Geometry check sheet. Reference: the model listing, model coordinates, mm. Face numbers are marked on the shaded views. A direction names the side the tool comes from. Round coordinates to 2 decimals unless told otherwise and drop trailing zeros. Write each loop counter-clockwise with the first axis right and the second up, starting at its lowest first coordinate (ties: lowest second). Pieces come first, ordered by that corner, then holes. Notation, with made-up numbers: M -14.75,5 L 23.25,5 A19 cw 23.25,25 Z; hole C 31,19.5 d9. An arc over 180 degrees is marked long. Use a Markdown table: item, result.
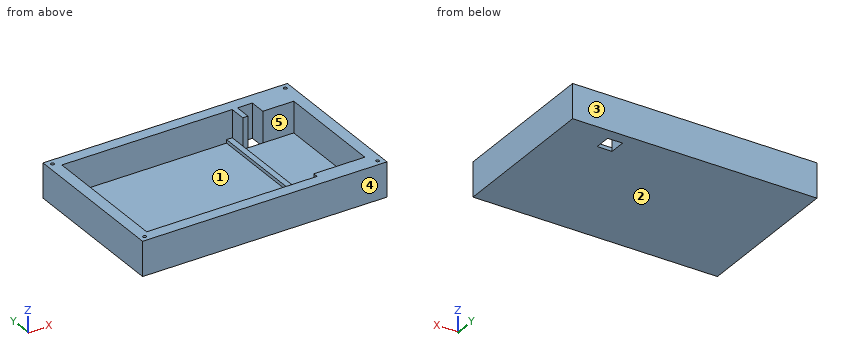
Autodesk Fusion 360 part; units mm, degrees
sketch "Sketch1" plane through (0, 0, 0) normal (0, 0, 1) x (1, 0, 0)
  line L0 (-50, 40) -> (143.2, 40)
  line L1 (143.2, 40) -> (143.2, -75.2)
  line L2 (143.2, -75.2) -> (-50, -75.2)
  line L3 (-50, -75.2) -> (-50, 40)
  line L4 (-60, 50) -> (153.2, 50)
  line L5 (153.2, 50) -> (153.2, -85.2)
  line L6 (153.2, -85.2) -> (-60, -85.2)
  line L7 (-60, -85.2) -> (-60, 50)
  circle A0 centre (-55, 45) radius 1.45
  circle A1 centre (148.2, 45) radius 1.45
  circle A2 centre (148.2, -80.2) radius 1.45
  circle A3 centre (-55, -80.2) radius 1.45
  line L8 (143.2, -75.2) -> (98.7, -75.2)
  line L9 (98.7, -75.2) -> (98.7, 21.3)
  line L10 (98.7, 21.3) -> (143.2, 21.3)
  line L11 (143.2, 21.3) -> (143.2, -75.2)
  line L12 (98.7, 21.3) -> (143.2, 21.3)
  line L13 (143.2, 21.3) -> (143.2, 40)
  line L14 (143.2, 40) -> (98.7, 40)
  line L15 (98.7, 40) -> (98.7, 21.3)
  line L16 (98.7, 40) -> (93.7, 40)
  line L17 (93.7, 40) -> (93.7, -75.2)
  line L18 (93.7, -75.2) -> (98.7, -75.2)
  line L19 (98.7, -75.2) -> (98.7, 40)
  dimension "d1" = 193.2
  dimension "d2" = 115.2
  dimension "d3" = 213.2
  dimension "d4" = 135.2
  dimension "d5" = 10
  dimension "d6" = 10
  dimension "d7" = 2.9
  dimension "d8" = 5
  dimension "d9" = 5
  dimension "d10" = 2.9
  dimension "d11" = 5
  dimension "d12" = 5
  dimension "d13" = 2.9
  dimension "d14" = 5
  dimension "d15" = 5
  dimension "d16" = 2.9
  dimension "d17" = 5
  dimension "d18" = 5
  dimension "d19" = 44.5
  dimension "d20" = 96.5
  dimension "d21" = 5
extrude "Extrude1" add sketch "Sketch1" along normal blind 3 contours L0 L2 L3 L17 | L1 L2 L8 L9 L10 L11 L12 L19 makes body 1 at (113.5333, -43.0333, 0) makes body 2 at (-2.1, 1.6, 0)
extrude "Extrude2" add sketch "Sketch1" along normal blind 6 contours L0 L2 L9 L15 L16 L17 L18 L19 bodies 1 2
extrude "Extrude3" add sketch "Sketch1" along normal blind 3 separate body contours A0 | A1 | A2 | A3 makes body 3 at (149.5361, -79.6368, 2) makes body 4 at (-54.0406, -79.1128, 2) makes body 5 at (149.3558, 45.8755, 2) makes body 6 at (-56.4213, 45.2873, 2)
extrude "Extrude4" add sketch "Sketch1" along normal blind 30 contours L0 L1 L10 L12 L13 L14 L15 L19 | L4 L5 L6 L7 bodies 1 3 4 5 6
sketch "Sketch2" plane through (0, 21.3, 0) normal (0, -1, 0) x (1, 0, 0)
  line L0 (98.7, 3) -> (143.2, 3)
  line L1 (143.2, 3) -> (143.2, 30)
  line L2 (143.2, 30) -> (98.7, 30)
  line L3 (98.7, 30) -> (98.7, 6)
  line L4 (98.7, 6) -> (98.7, 3)
  line L5 (103.2, 30) -> (116.2, 30)
  line L6 (116.2, 30) -> (116.2, 3)
  line L7 (116.2, 3) -> (103.2, 3)
  line L8 (103.2, 3) -> (103.2, 30)
  dimension "d30" = 13
  dimension "d32" = 4.5
extrude "Extrude5" cut sketch "Sketch2" against normal blind 18.7 contours L0 L2 L5 L6 L7 L8 bodies 1
sketch "Sketch3" plane through (0, 0, 3) normal (0, 0, 1) x (-1, 0, 0)
  line L0 (-98.7, 75.2) -> (-143.2, 75.2)
  line L1 (-143.2, 75.2) -> (-143.2, -21.3)
  line L2 (-143.2, -21.3) -> (-116.2, -21.3)
  line L3 (-116.2, -21.3) -> (-116.2, -40)
  line L4 (-116.2, -40) -> (-103.2, -40)
  line L5 (-103.2, -40) -> (-103.2, -21.3)
  line L6 (-103.2, -21.3) -> (-98.7, -21.3)
  line L7 (-98.7, -21.3) -> (-98.7, 75.2)
  line L8 (-103.2, -40) -> (-116.2, -40)
  line L9 (-116.2, -40) -> (-116.2, -21.3)
  line L10 (-116.2, -21.3) -> (-103.2, -21.3)
  line L11 (-103.2, -21.3) -> (-103.2, -40)
extrude "Extrude6" cut sketch "Sketch3" against normal blind 6 contours L3 L4 L5 L8 L9 L10 L11 bodies 1
sketch "Sketch4" plane through (0, -75.2, 0) normal (0, 1, 0) x (-1, 0, 0)
  line L0 (-143.2, 3) -> (-98.7, 3)
  line L1 (-98.7, 3) -> (-98.7, 6)
  line L2 (-98.7, 6) -> (-93.7, 6)
  line L3 (-93.7, 6) -> (-93.7, 3)
  line L4 (-93.7, 3) -> (50, 3)
  line L5 (50, 3) -> (50, 30)
  line L6 (50, 30) -> (-143.2, 30)
  line L7 (-143.2, 30) -> (-143.2, 3)
  line L8 (-98.7, 3) -> (-143.2, 3)
  line L9 (-143.2, 3) -> (-143.2, 30)
  line L10 (-143.2, 30) -> (-98.7, 30)
  line L11 (-98.7, 30) -> (-98.7, 3)
extrude "Extrude7" add sketch "Sketch4" along normal blind 4.5 contours L0 L1 L6 L7 L8 L9 L10 L11 bodies 1
extrude "Extrude8" cut 2 faces at (101.7, 21.3, 13) (125.2, 21.3, 12) along direction (0, 1, 0) blind 4.5 on bodies 1 bodies 1
extrude "Extrude9" add 1 faces at (111.8667, 21.3, 2) along direction (0, 1, 0) blind 4.5 on bodies 1 bodies 1
equation "d3 = 193.2 mm + 20 mm"
equation "d4 = 115.2 mm + 20 mm"
Item 1: Cross-section at A-A, the plane y = 37. Record the cut outline in (x, z).
Outcome:
| item | result |
|---|---|
| outline | M -60,0 L 103.2,0 L 103.2,30 L 98.7,30 L 98.7,6 L 93.7,6 L 93.7,3 L -50,3 L -50,30 L -60,30 Z; M 116.2,0 L 153.2,0 L 153.2,30 L 116.2,30 Z |
Item 2: Cross-section at C-C, the plane z = 13. Record the cut outline in (x, y), and give its area (3 significant figures).
Outcome:
| item | result |
|---|---|
| outline | M -60,-85.2 L 153.2,-85.2 L 153.2,50 L -60,50 Z; hole C -55,-80.2 d2.9; hole C -55,45 d2.9; hole M -50,-75.2 L 98.7,-75.2 L 98.7,-70.7 L 143.2,-70.7 L 143.2,25.8 L 116.2,25.8 L 116.2,40 L 103.2,40 L 103.2,25.8 L 98.7,25.8 L 98.7,40 L -50,40 Z; hole C 148.2,-80.2 d2.9; hole C 148.2,45 d2.9 |
| area | 7,190 mm2 |
Item 3: Cross-section at B-B, the plane x = 96. Record the cut outline in (y, z).
Outcome:
| item | result |
|---|---|
| outline | M -85.2,0 L 50,0 L 50,30 L 40,30 L 40,6 L -75.2,6 L -75.2,30 L -85.2,30 Z |
Item 4: Access from +Z, -Z, +X, -X, +Y, -Y to the whole of each face (thin tool, end or side, straight path). Record for the marked faces 1 and 2.
Outcome:
| item | result |
|---|---|
| face 1 | +Z |
| face 2 | -Z, +X, -X, +Y, -Y |
Item 5: Mould release check, pull along Y, two halves, no side actions. Record for the marked faces 3, 4 and 5: +Y half, -Y half, draft (parallel to the pull), parting line (faces both ways), or undercut.
Outcome:
| item | result |
|---|---|
| face 3 | +Y half |
| face 4 | -Y half |
| face 5 | undercut |
Item 6: Go/stop test with flat-tipped pins: pin 1 (4 mm diameter, centred on x = 44, y = -41, fed in from +Z); pin 2 (4 mm diameter, centred on x = 96.5, y = 3.5, fed in from +Z). Record where each tip stops, or that it passes through.
Outcome:
| item | result |
|---|---|
| pin 1 | stops at z = 3 |
| pin 2 | stops at z = 6 |
Item 7: Cross-section at D-D, the plane y = -66. Record the cut outline in (x, z), and give its area (3 significant figures).
Outcome:
| item | result |
|---|---|
| outline | M -60,0 L 153.2,0 L 153.2,30 L 143.2,30 L 143.2,3 L 98.7,3 L 98.7,6 L 93.7,6 L 93.7,3 L -50,3 L -50,30 L -60,30 Z |
| area | 1,190 mm2 |
Item 8: Material ranges on line 1 along X through (y, z) = (27, 20.5); line 2 along X through (y, z) = (-80.2, 11.5); line 3 along Y through (x, z) = (148.2, 9), recorded low to high. Write a range as from..to.
Outcome:
| item | result |
|---|---|
| line 1 | x = -60..-50, 98.7..103.2, 116.2..153.2 |
| line 2 | x = -60..-56.45, -53.55..146.75, 149.65..153.2 |
| line 3 | y = -85.2..-81.65, -78.75..43.55, 46.45..50 |
